from build123d import *

# Parameters (mm, degrees)
SKETCH1_W                      = 35
SKETCH1_H                      = 30
BOSS_EXTRUDE1_DEPTH            = 20
M4X0_7_TAPPED_HOLE1_AT_2_COUNT = 2
M4X0_7_TAPPED_HOLE1_AT_2_PITCH = 18.027756377
M4X0_7_TAPPED_HOLE1_AT_3_COUNT = 2
M4X0_7_TAPPED_HOLE1_AT_3_PITCH = 15
M4X0_7_TAPPED_HOLE1_AT_4_COUNT = 2
M4X0_7_TAPPED_HOLE1_AT_4_PITCH = 10


with BuildPart() as part:
    # Sketch1 → Boss-Extrude1 (new body)
    with BuildSketch(Plane.XY):
        with Locations((-17.5, 15)):
            Rectangle(SKETCH1_W, SKETCH1_H)
    extrude(amount=BOSS_EXTRUDE1_DEPTH)

    # Sketch6 → M4x0.7 Tapped Hole1 (revolve, cut)
    with BuildSketch(Plane(origin=(-35, 21.5125, 5), x_dir=(0, 0, 1), z_dir=(0, 1, 0))):
        Polygon((0, 0), (0, 14.491420021), (1.65, 13.5), (1.65, 0), align=None)
    m4x0_7_tapped_hole1 = revolve(axis=Axis((-41.35, 21.5125, 5), (1, 0, 0)), mode=Mode.SUBTRACT)

    # M4x0.7 Tapped Hole1 at 2: M4x0.7 Tapped Hole1 ×2
    with Locations(*[Vector(0, -0.832050294, 0.554700196) * (i * M4X0_7_TAPPED_HOLE1_AT_2_PITCH) for i in range(1, M4X0_7_TAPPED_HOLE1_AT_2_COUNT)]):
        add(m4x0_7_tapped_hole1, mode=Mode.SUBTRACT)

    # M4x0.7 Tapped Hole1 at 3: M4x0.7 Tapped Hole1 ×2
    with Locations(*[(0, -i * M4X0_7_TAPPED_HOLE1_AT_3_PITCH, 0) for i in range(1, M4X0_7_TAPPED_HOLE1_AT_3_COUNT)]):
        add(m4x0_7_tapped_hole1, mode=Mode.SUBTRACT)

    # M4x0.7 Tapped Hole1 at 4: M4x0.7 Tapped Hole1 ×2
    with Locations(*[(0, 0, i * M4X0_7_TAPPED_HOLE1_AT_4_PITCH) for i in range(1, M4X0_7_TAPPED_HOLE1_AT_4_COUNT)]):
        add(m4x0_7_tapped_hole1, mode=Mode.SUBTRACT)

    # Mirror1: M4x0.7 Tapped Hole1 across plane
    add(m4x0_7_tapped_hole1.mirror(Plane.ZY.offset(17.5)), mode=Mode.SUBTRACT)

    # Mirror1 copy 1 sketch → Mirror1 copy 1 (revolve, cut)
    with BuildSketch(Plane(origin=(0, 6.5125, 15), x_dir=(0, 0, 1), z_dir=(0, 1, 0))):
        Polygon((0, 0), (0, -14.491420021), (1.65, -13.5), (1.65, 0), align=None)
    revolve(axis=Axis((6.35, 6.5125, 15), (1, 0, 0)), mode=Mode.SUBTRACT)

    # Mirror1 copy 2 sketch → Mirror1 copy 2 (revolve, cut)
    with BuildSketch(Plane(origin=(0, 6.5125, 5), x_dir=(0, 0, 1), z_dir=(0, 1, 0))):
        Polygon((0, 0), (0, -14.491420021), (1.65, -13.5), (1.65, 0), align=None)
    revolve(axis=Axis((6.35, 6.5125, 5), (1, 0, 0)), mode=Mode.SUBTRACT)

    # Mirror1 copy 3 sketch → Mirror1 copy 3 (revolve, cut)
    with BuildSketch(Plane(origin=(0, 21.5125, 15), x_dir=(0, 0, 1), z_dir=(0, 1, 0))):
        Polygon((0, 0), (0, -14.491420021), (1.65, -13.5), (1.65, 0), align=None)
    revolve(axis=Axis((6.35, 21.5125, 15), (1, 0, 0)), mode=Mode.SUBTRACT)


solid = part.part
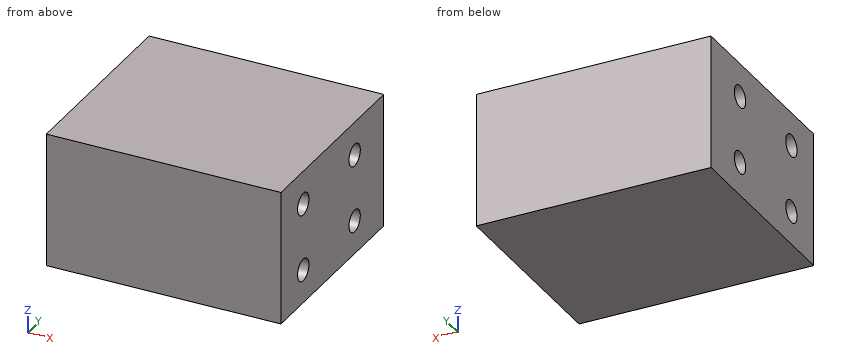
The listing builds one solid part. Answer for the finished solid, in the listing's coordinates (mm). Round coordinates to 2 decimals unless told otherwise and drop trailing zeros. Order: outer loops, then holes, each group sorted by start corner. A loop starts at its lowest first (then second) coordinate and runs counter-clockwise, first axis right, second up. Notation, with made-up numbers: (-7.5, -2.5) -> (18.5, -2.5) arc R17 ccw to (18.5, 20.5) -> close; hole circle Ø4 at (53.5, 71.5). An arc over 180 degrees is marked (long way). One line per item, written item: value.
Item 1: Straight lines are drawn through the part: L1, parallel to Y at x = -2.75, z = 5; L2, parallel to Z at x = -10.5, y = 22.25; L3, parallel to Y at x = -22, z = 5.25. For each, find the intervals that lie inside material, in ascending order.
Taken from the geometry:
L1: y = 0 to 4.86, 8.16 to 19.86, 23.16 to 30
L2: z = 0 to 3.52, 6.48 to 13.52, 16.48 to 20
L3: y = 0 to 4.88, 8.14 to 19.88, 23.14 to 30
Item 2: Find section A-A, the plane x = -4. Give the vertices of the cut face in (y, z).
Taken from the geometry:
outline: (0, 0) -> (30, 0) -> (30, 20) -> (0, 20) -> close; hole circle Ø3.3 at (6.51, 5); hole circle Ø3.3 at (6.51, 15); hole circle Ø3.3 at (21.51, 5); hole circle Ø3.3 at (21.51, 15)
Item 3: Given P1, Ø2.5, axis at y = 21.51, z = 15, coming from the -X side; P2, Ø2.5, axis at y = 21.51, z = 5, coming from the +X side, each flat-ended and moving along its own axis, determine where each tip first touches the part or whether it passes through.
Taken from the geometry:
P1: stops at x = -21.26
P2: stops at x = -13.74
